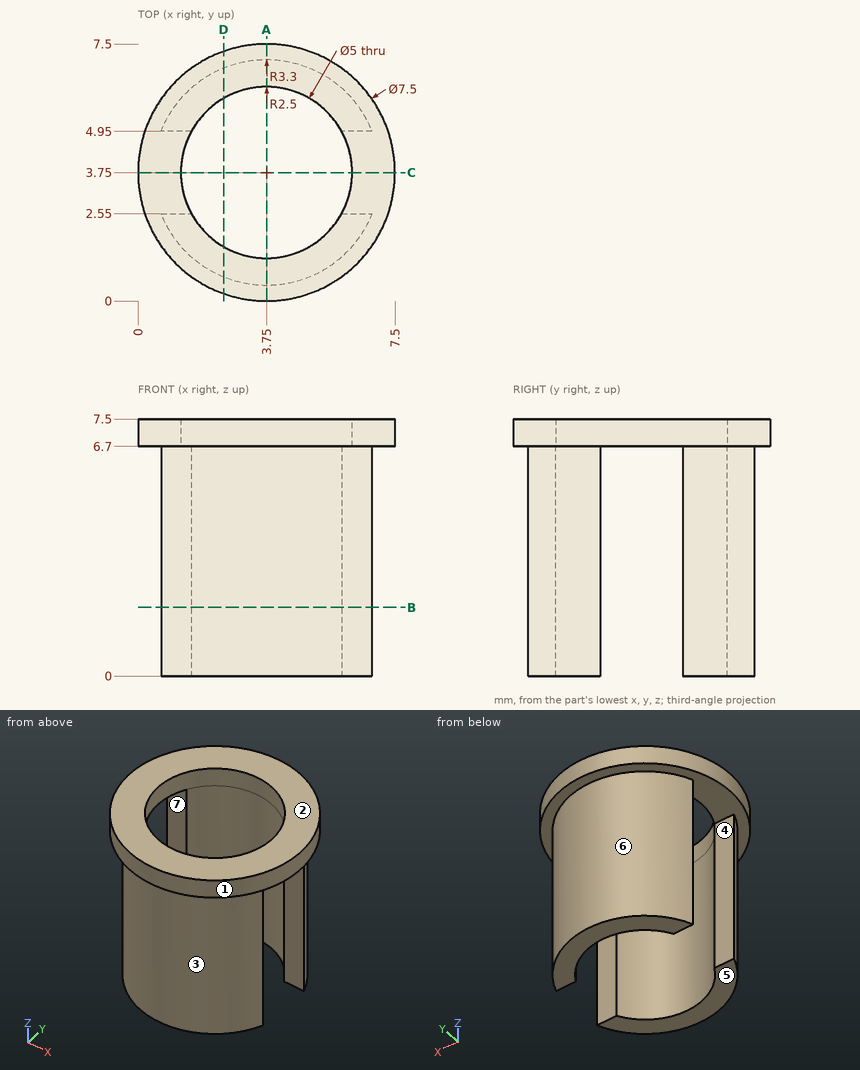
Answer from the drawing. Dimensions are ordinates in mm from the lowest x, y and z of the part. A direction names the side the tool comes from. Coordinates: 2 decimals unless noted, no trailing zeros. Loops run counter-clockwise (first coordinate to the right, second up) from the corner with the lowest first, then second, coordinate; pieces in that order, holes last. Notation, with made-up numbers: (-7, 63.5) - (-3, 63.5) arc R20 cw to (-3, 81.5) - close; hole circle Ø4 at (38, 74). An arc over 180 degrees is marked (long way). Answer in a Markdown table with one row per item.
1. Determine the mould class of the marked faces 1, 2, 3 and 4 for opening direction Y: +Y half, -Y half, draft (parallel to the pull), parting line (faces both ways), or undercut.
Conclusion:
| item | result |
|---|---|
| face 1 | parting line |
| face 2 | draft |
| face 3 | -Y half |
| face 4 | undercut |
2. Find section D-D, the plane x = 2.5. Write down the section's boundary in (y, z).
Conclusion:
| item | result |
|---|---|
| outline | (0.21, 6.7) - (0.7, 6.7) - (0.7, 0) - (1.58, 0) - (1.58, 7.5) - (0.21, 7.5) - close; (5.92, 0) - (6.8, 0) - (6.8, 6.7) - (7.29, 6.7) - (7.29, 7.5) - (5.92, 7.5) - close |
3. Find section A-A, the plane x = 3.75. Write down the section's boundary in (y, z), then the cut area to 3 significant figures.
Conclusion:
| item | result |
|---|---|
| outline | (0, 6.7) - (0.45, 6.7) - (0.45, 0) - (1.25, 0) - (1.25, 7.5) - (0, 7.5) - close; (6.25, 0) - (7.05, 0) - (7.05, 6.7) - (7.5, 6.7) - (7.5, 7.5) - (6.25, 7.5) - close |
| area | 12.7 mm² |
4. Which of the six approach directions +Z, -Z, +X, -X, +Y, -Y give full straight-line access (tool end or side, diameter ignored) to the marked faces 5, 6 and 7?
Conclusion:
| item | result |
|---|---|
| face 5 | -Z, +X, -X, +Y, -Y |
| face 6 | -Z, +Y |
| face 7 | -Z, +X, -X |
5. Given pin 1 (0.7 mm diameter, centred on x = 6.5, z = 2.5, fed in from -Y); pin 2 (1 mm diameter, centred on x = 1, z = 6, fed in from +Y); pin 3 (0.7 mm diameter, centred on x = 1.5, z = 4.5, fed in from +Y), each flat-ended and moving along its own axis, determine where each tip first touches the part or whether it passes through.
Conclusion:
| item | result |
|---|---|
| pin 1 | stops at y = 1.49 |
| pin 2 | stops at y = 6.16 |
| pin 3 | stops at y = 6.45 |
6. Straight lines are drawn through the part: line 1 (Y direction, x = 3.75, z = 6.9); line 2 (Y direction, x = 5.75, z = 1.25); line 3 (Z direction, x = 2.75, y = 7). For each, find the intervals that lie inside material, in ascending order.
Conclusion:
| item | result |
|---|---|
| line 1 | y = 0 to 1.25, 6.25 to 7.5 |
| line 2 | y = 1.13 to 2.25, 5.25 to 6.37 |
| line 3 | z = 6.7 to 7.5 |
7. Find section C-C, the plane y = 3.75. Write down the section's boundary in (x, z).
Conclusion:
| item | result |
|---|---|
| outline | (0, 6.7) - (1.25, 6.7) - (1.25, 7.5) - (0, 7.5) - close; (6.25, 6.7) - (7.5, 6.7) - (7.5, 7.5) - (6.25, 7.5) - close |
8. Find section B-B, the plane z = 2. Write down the section's boundary in (x, y).
Conclusion:
| item | result |
|---|---|
| outline | (0.68, 2.55) arc R3.3 ccw to (6.82, 2.55) - (5.94, 2.55) arc R2.5 cw to (1.56, 2.55) - close; (0.68, 4.95) - (1.56, 4.95) arc R2.5 cw to (5.94, 4.95) - (6.82, 4.95) arc R3.3 ccw to start |
